from build123d import *

# Parameters (mm, degrees)
CROQUIS1_W              = 15
CROQUIS1_H              = 3
CROQUIS1_W_2            = 5
CROQUIS1_W_3            = 30
CROQUIS1_H_2            = 9
SALIENTE_EXTRUIR1_DEPTH = 3
CROQUIS3_W              = 3
CROQUIS3_H              = 7
CROQUIS3_W_2            = 7
CROQUIS3_H_2            = 3
CORTAR_EXTRUIR2_DEPTH   = 4
CORTAR_EXTRUIR3_DEPTH   = 4
CORTAR_EXTRUIR4_DEPTH   = 4
CROQUIS7_W              = 10
CROQUIS7_H              = 3
CORTAR_EXTRUIR5_DEPTH   = 4


with BuildPart() as part:
    # Croquis1 → Saliente-Extruir1 (new body)
    with BuildSketch(Plane.XY):
        with BuildLine():
            Line((0, 0), (15, 0))
            Line((15, 0), (15, 12))
            ThreePointArc((15, 12), (30, 27), (45, 12))
            Line((45, 12), (45, 0))
            Line((45, 0), (120, 0))
            Line((120, 0), (78.045018441, 50))
            Line((78.045018441, 50), (15, 50))
            Line((15, 50), (0, 0))
        make_face()
        with Locations((97.5, 3.5)):
            Rectangle(CROQUIS1_W, CROQUIS1_H, mode=Mode.SUBTRACT)
        with Locations((67.5, 3.5)):
            Rectangle(CROQUIS1_W, CROQUIS1_H, mode=Mode.SUBTRACT)
        with Locations((7.5, 3.5)):
            Rectangle(CROQUIS1_W_2, CROQUIS1_H, mode=Mode.SUBTRACT)
        with Locations((67, 12.5)):
            Rectangle(CROQUIS1_W_3, CROQUIS1_H_2, mode=Mode.SUBTRACT)
    extrude(amount=SALIENTE_EXTRUIR1_DEPTH)

    # Croquis3 → Cortar-Extruir2 (cut, through all)
    with BuildSketch(Plane.XY.offset(3)):
        with Locations((76.545018441, 36.5)):
            Rectangle(CROQUIS3_W, CROQUIS3_H)
        with Locations((84.545018441, 26.5)):
            Rectangle(CROQUIS3_W_2, CROQUIS3_H_2)
    extrude(amount=-CORTAR_EXTRUIR2_DEPTH, mode=Mode.SUBTRACT)

    # Croquis5 → Cortar-Extruir3 (cut, through all)
    with BuildSketch(Plane.XY.offset(3)):
        Polygon((103.563039053, 19.58880726), (101.264905723, 17.660444431), (107.69278182, 10), (109.99091515, 11.928362829), align=None)
    extrude(amount=-CORTAR_EXTRUIR3_DEPTH, mode=Mode.SUBTRACT)

    # Croquis6 → Cortar-Extruir4 (cut, through all)
    with BuildSketch(Plane.XY.offset(3)):
        Polygon((8.532091953, 28.440306509), (11.405570808, 27.578262852), (8.532091953, 18), (5.658613097, 18.862043657), align=None)
    extrude(amount=-CORTAR_EXTRUIR4_DEPTH, mode=Mode.SUBTRACT)

    # Croquis7 → Cortar-Extruir5 (cut, through all)
    with BuildSketch(Plane(origin=(0, 0, 0), x_dir=(-1, 0, 0), z_dir=(0, 0, -1))):
        with Locations((-57.545018441, 46.5)):
            Rectangle(CROQUIS7_W, CROQUIS7_H)
        with Locations((-32.545018441, 46.5)):
            Rectangle(CROQUIS7_W, CROQUIS7_H)
    extrude(amount=-CORTAR_EXTRUIR5_DEPTH, mode=Mode.SUBTRACT)


solid = part.part
Could you check a few things on this model? Use its own coordinates, in mm. A direction names the side the tool comes from. Coordinates: 2 decimals unless noted, no trailing zeros. Order: outer loops, then holes, each group sorted by start corner. A loop starts at its lowest first (then second) coordinate and runs counter-clockwise, first axis right, second up.
Q1. Will these pins go through, and if not, where does the flat tip stop? pin 1 (1.5 mm diameter, centred on y = 10.5, z = 1.5, fed in from -X) (3 decimals); pin 2 (1.5 mm diameter, centred on y = 35, z = 1.5, fed in from +X); pin 3 (1 mm diameter, centred on y = 6, z = 0.5, fed in from +X).
Q2. Suppose I cut it at B-B on x = 30. Please give me the cut outline in (y, z), and give its area (3 significant figures).
Q3. Thinking about a two-plate mould opening in Y: for faces 4 (the flat face through (52.545, 46, 1)), 5 (the flat face through (15, 6, 1)), 6 (the flat face through (47, 50, 1)), which applies, released by +Y, released by -Y, zero draft, split by the parting line, or undercut?
Q4. Suppose I cut it at C-C on z = 2.55. Give the number of separate pieces and of enclosed holes in the cut face, and give its area (3 significant figures).
Q5. Which directions (+Z, -Z, +X, -X, +Y, -Y) give clear straight access to the entire face, cutting with the end or side of a thin tool? Please do faces 1 (the flat face through (81.045, 26, 2)), 2 (the flat face through (45, 6, 1)), 3 (the flat face through (10, 28, 2)).
Q6. Suppose I cut it at A-A on x = 68.5. Please give me the cut outline in (y, z).
Q7. Suppose I cut it at D-D on x = 106.5. Please give me the cut outline in (y, z), and give its area (3 significant figures).
Q8. Please list where these lines run through material, in increasing order: L1, parallel to Y at x = 75.5, z = 1; L2, parallel to Y at x = 63, z = 0.85; L3, parallel to X at y = 12.5, z = 2.55.
Answer:
1. pin 1: stops at x = 2.925
1. pin 2: stops at x = 91.26
1. pin 3: stops at x = 115.38
2. outline: (27, 0) - (45, 0) - (45, 3) - (27, 3) - close; (48, 0) - (50, 0) - (50, 3) - (48, 3) - close
2. area: 60.0 mm2
3. face 4: undercut
3. face 5: zero draft
3. face 6: released by +Y
4. separate pieces: 1
4. enclosed holes: 8
4. area: 3,330 mm2
5. face 1: +Z, -Z
5. face 2: +Z, -Z, -Y
5. face 3: +Z, -Z, -X
6. outline: (0, 0) - (2, 0) - (2, 3) - (0, 3) - close; (5, 0) - (8, 0) - (8, 3) - (5, 3) - close; (17, 0) - (50, 0) - (50, 3) - (17, 3) - close
7. outline: (0, 0) - (11.42, 0) - (11.42, 3) - (0, 3) - close
7. area: 34.3 mm2
8. L1: y = 0 to 8, 17 to 33, 40 to 50
8. L2: y = 0 to 2, 5 to 8, 17 to 50
8. L3: x = 3.75 to 15.01, 44.99 to 52, 82 to 105.6
